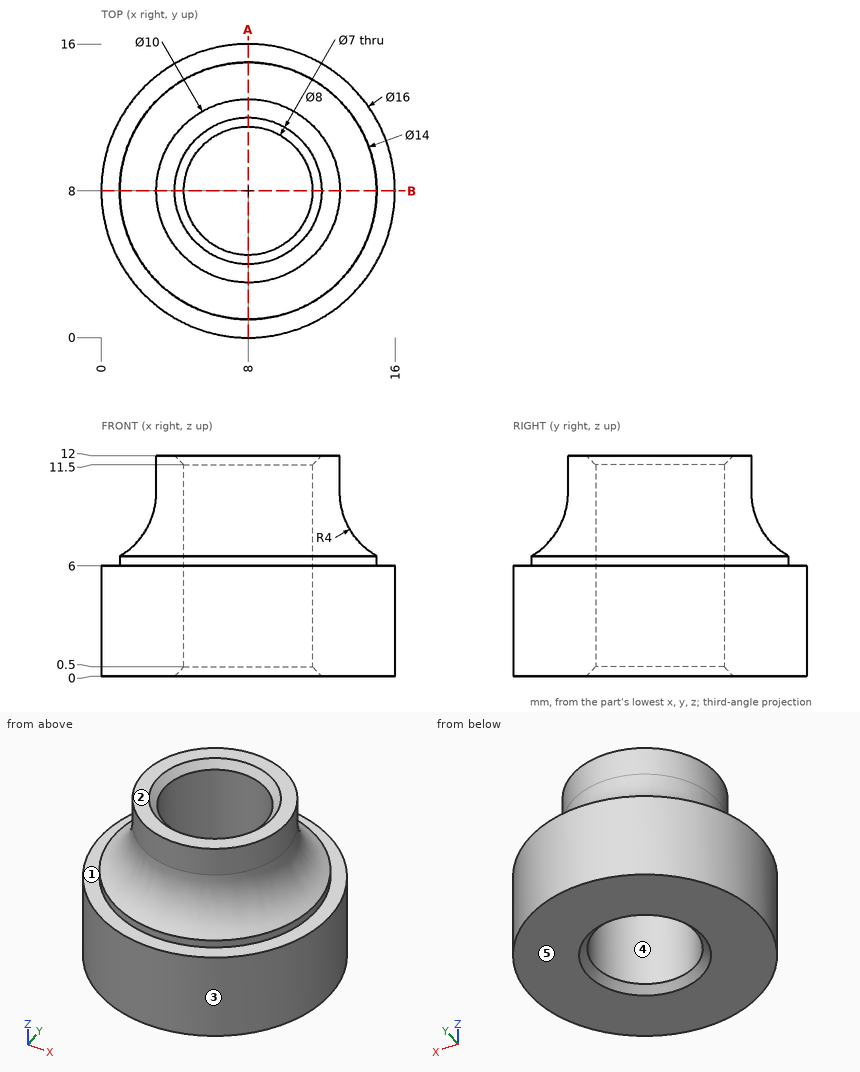
Could you check a few things on this drawing? It's one solid part, dimensions in mm from its lowest x, y, z. A direction names the side the tool comes from. Coordinates: 2 decimals unless noted, no trailing zeros. Order: outer loops, then holes, each group sorted by start corner. A loop starts at its lowest first (then second) coordinate and runs counter-clockwise, first axis right, second up. Notation, with made-up numbers: (-10, 23) - (9, 23) arc R14 cw to (9, 44) - close; hole circle Ø11 at (-18.75, 51). An arc over 180 degrees is marked (long way). One line per question, with ' | ' between items.
(1) If I drill on L1, parallel to Y at x = 8, z = 5.5; L2, parallel to X at y = 6.25, z = 5; L3, parallel to Y at x = 8, z = 8.5, over which ranges is the centre line in solid material (lowest first)?
Report:
L1: y = 0 to 4.5, 11.5 to 16 | L2: x = 0.19 to 4.97, 11.03 to 15.81 | L3: y = 2.71 to 4.5, 11.5 to 13.29
(2) If we mould it in two halves opening along Y, with no side actions, what happens to the marked faces 3, 4 and 5? For each: pulls with the +Y half, pulls with the -Y half, needs draft (parallel to the pull), parting line crosses it, or undercut.
Report:
face 3: parting line crosses it | face 4: undercut | face 5: needs draft
(3) Suppose I cut it at A-A on x = 8. List the corners of the cut face in (y, z) for me.
Report:
outline: (0, 0) - (4, 0) - (4.5, 0.5) - (4.5, 11.5) - (4, 12) - (3, 12) - (3, 10) arc R4 cw to (1, 6.54) - (1, 6) - (0, 6) - close; (11.5, 0.5) - (12, 0) - (16, 0) - (16, 6) - (15, 6) - (15, 6.54) arc R4 cw to (13, 10) - (13, 12) - (12, 12) - (11.5, 11.5) - close
(4) For the marked faces 1 and 2, which set-ups out of +Z, -Z, +X, -X, +Y, -Y let a thin tool reach every point of the face, with its end or its side?
Report:
face 1: +Z | face 2: +Z, +X, -X, +Y, -Y
(5) Will these pins go through, and if not, where does the flat tip stop? pin 1 (6.5 mm diameter, centred on x = 8, y = 8, fed in from -Z); pin 2 (1 mm diameter, centred on x = 9, z = 5.5, fed in from +Y); pin 3 (5 mm diameter, centred on y = 7, z = 5.5, fed in from +X); pin 4 (6 mm diameter, centred on x = 2, z = 4, fed in from -Y).
Report:
pin 1: passes through | pin 2: stops at y = 15.98 | pin 3: stops at x = 16 | pin 4: stops at y = 0.58
